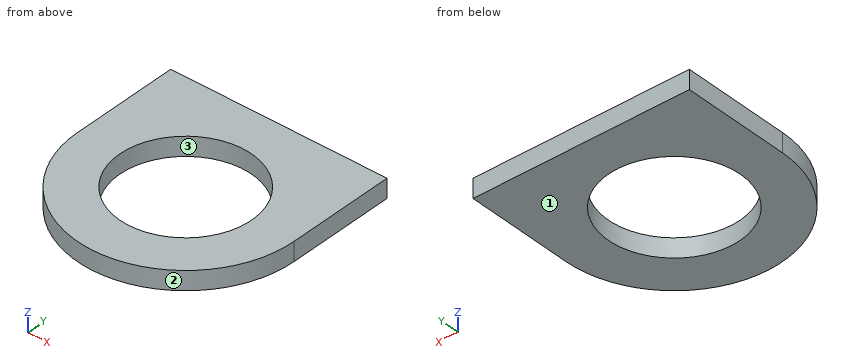
```python
from build123d import *

# Parameters (mm, degrees)
SKETCH1_R           = 1.7399
BOSS_EXTRUDE1_DEPTH = 0.5


with BuildPart() as part:
    # Sketch1 → Boss-Extrude1 (new body)
    with BuildSketch(Plane(origin=(0, 0, 764.167404568), x_dir=(-1, 0, 0), z_dir=(0, 0, -1))):
        with BuildLine():
            Line((108.204437713, 637.468625119), (108.204437713, 640.326125119))
            Line((108.204437713, 640.326125119), (111.061937713, 640.326125119))
            Line((111.061937713, 640.326125119), (113.919437713, 640.326125119))
            Line((113.919437713, 640.326125119), (113.919437713, 637.468625119))
            ThreePointArc((113.919437713, 637.468625119), (111.061937713, 634.611125119), (108.204437713, 637.468625119))
        make_face()
        with Locations((111.061937713, 637.468625119)):
            Circle(SKETCH1_R, mode=Mode.SUBTRACT)
    extrude(amount=BOSS_EXTRUDE1_DEPTH)


solid = part.part
```
For this review, take the finished solid that the model builds, in its own axes (mm). Face numbers are marked on the shaded views. Round coordinates to 2 decimals unless told otherwise and drop trailing zeros. Write each loop counter-clockwise with the first axis right and the second up, starting at its lowest first coordinate (ties: lowest second). Pieces come first, ordered by that corner, then holes. Notation, with made-up numbers: M 0.5,-35 L 20.5,-35 A7 ccw 20.5,-22 Z; hole C 41.5,-14.75 d8. An arc over 180 degrees is marked long. One line per item, written item: value. Start each with the question number.
(1) We need section C-C (y = 636.15). Give the boundary of the cut face in (x, z).
(2) We need section A-A (z = 764). Give the boundary of the cut face in (x, y) (1 decimal).
(3) Wall thickness on line 1 (Y direction, x = -109.9, z = 763.9); line 2 (X direction, y = 638, z = 764.05); line 3 (X direction, y = 636.2, z = 764): over which ranges is each line inside the solid? List them lowest first.
(4) We need section B-B (x = -109.85). Give the boundary of the cut face in (y, z).
(5) We need section D-D (y = 635.3). Give the boundary of the cut face in (x, z), and give its area (3 significant figures).
(6) The part is to be moulded in two halves that separate along X. For the marked faces 1, 2 and 3, say which applies: released by +X, released by -X, zero draft, split by the parting line, or undercut.
Result:
1. outline: M -113.6,763.67 L -112.2,763.67 L -112.2,764.17 L -113.6,764.17 Z; M -109.93,763.67 L -108.53,763.67 L -108.53,764.17 L -109.93,764.17 Z
2. outline: M -113.9,637.5 A2.9 ccw -108.2,637.5 L -108.2,640.3 L -113.9,640.3 Z; hole C -111.1,637.5 d3.5
3. line 1: 634.86 to 636.17, 638.76 to 640.33
3. line 2: -113.92 to -112.72, -109.41 to -108.2
3. line 3: -113.62 to -112.25, -109.87 to -108.5
4. outline: M 634.88,763.67 L 636.22,763.67 L 636.22,764.17 L 634.88,764.17 Z; M 638.72,763.67 L 640.33,763.67 L 640.33,764.17 L 638.72,764.17 Z
5. outline: M -112.92,763.67 L -109.2,763.67 L -109.2,764.17 L -112.92,764.17 Z
5. area: 1.86 mm²
6. face 1: zero draft
6. face 2: split by the parting line
6. face 3: undercut
